The model under review builds one solid part; all positions refer to its coordinate system, in mm. Give positions to 0.01 mm unless a question says otherwise; leave off trailing zeros. Write each loop counter-clockwise with the first axis right and the second up, starting at its lowest first coordinate (ties: lowest second). Pieces come first, ordered by that corner, then holes. Notation, with made-up numbers: (17.25, 0.5) -> (47.25, 0.5) arc R17 cw to (47.25, 13.5) -> close; hole circle Ø9 at (13.5, 22). An arc over 180 degrees is marked (long way). Use CSV: the item, a comma, the result in double quotes.
```python
from build123d import *

# Parameters (mm, degrees)
EXTRUDE_1_DEPTH     = 3
SKETCH_4_R          = 1.5
CUT_EXTRUDE_2_DEPTH = 5
SKETCH_6_R          = 1.5
CUT_EXTRUDE_4_DEPTH = 5
SKETCH_7_W          = 3
SKETCH_7_H          = 15
CUT_EXTRUDE_5_DEPTH = 10


with BuildPart() as part:
    # 草图2 → 凸台-拉伸1 (new body)
    with BuildSketch(Plane.XY):
        Polygon((-7.5, 56.5), (-7.5, 55.5), (7.5, 55.5), (7.5, 56.5), (12, 56.5), (12, 48.5), (100, 5), (100, -20), (-100, -20), (-100, 5), (-12, 48.5), (-12, 56.5), align=None)
    extrude(amount=EXTRUDE_1_DEPTH)

    # 草图4 → 切除-拉伸2 (cut)
    with BuildSketch(Plane.XY.offset(3)):
        with Locations((-5, -5)):
            Circle(SKETCH_4_R)
        with Locations((5, -5)):
            Circle(SKETCH_4_R)
        with Locations((-5, -15)):
            Circle(SKETCH_4_R)
        with Locations((5, -15)):
            Circle(SKETCH_4_R)
    extrude(amount=-CUT_EXTRUDE_2_DEPTH, mode=Mode.SUBTRACT)

    # 草图6 → 切除-拉伸4 (cut)
    with BuildSketch(Plane.XY.offset(3)):
        with Locations((-9, 45.5)):
            Circle(SKETCH_6_R)
        with Locations((9, 45.5)):
            Circle(SKETCH_6_R)
    extrude(amount=-CUT_EXTRUDE_4_DEPTH, mode=Mode.SUBTRACT)

    # 草图7 → 切除-拉伸5 (cut)
    with BuildSketch(Plane.XY.offset(3)):
        with Locations((-58.5, 9.5)):
            Rectangle(SKETCH_7_W, SKETCH_7_H)
        with Locations((58.5, 9.5)):
            Rectangle(SKETCH_7_W, SKETCH_7_H)
    extrude(amount=-CUT_EXTRUDE_5_DEPTH, mode=Mode.SUBTRACT)


solid = part.part
```
Q1. Consider section A-A (z = 1.9). State how many separate pieces and enclosed holes the cut face has, then the cut area to 3 significant figures.
Derived:
separate pieces,"1"
enclosed holes,"8"
area,"9,920 mm2"
Q2. Insertion check: pin 1 (1.8 mm diameter, centred on x = -9, y = 45.5, fed in from -Z); pin 2 (1.5 mm diameter, centred on x = -1.5, z = 1.5, fed in from +Y); pin 3 (1.5 mm diameter, centred on y = 8.5, z = 2, fed in from -X); pin 4 (1.5 mm diameter, centred on y = 51, z = 1, fed in from -X). Each pin has a flat end and moves straight along its axis. Give the tip position at first contact, or say it passes through.
Derived:
pin 1,"passes through"
pin 2,"stops at y = 55.5"
pin 3,"stops at x = -94.44"
pin 4,"stops at x = -12"
Q3. Consider section B-B (y = 13.5). Write out the cut boundary in (x, z).
Derived:
outline,"(-82.8, 0) -> (-60, 0) -> (-60, 3) -> (-82.8, 3) -> close; (-57, 0) -> (57, 0) -> (57, 3) -> (-57, 3) -> close; (60, 0) -> (82.8, 0) -> (82.8, 3) -> (60, 3) -> close"
Q4. Consider section C-C (x = 71.5). Write out the cut boundary in (y, z), then the cut area to 3 significant figures.
Derived:
outline,"(-20, 0) -> (19.09, 0) -> (19.09, 3) -> (-20, 3) -> close"
area,"117 mm2"
Q5. To check wall thickness, follow probe 1 along Y at (x, z) = (-5, 1.75); probe 2 along X at (y, z) = (4, 2); probe 3 along X at (y, z) = (-14, 1.6). State the ranges of each line that lie inside material, in increasing order.
Derived:
probe 1,"y = -20 to -16.5, -13.5 to -6.5, -3.5 to 55.5"
probe 2,"x = -100 to -60, -57 to 57, 60 to 100"
probe 3,"x = -100 to -6.12, -3.88 to 3.88, 6.12 to 100"
Q6. Consider section D-D (x = -74). Write out the cut boundary in (y, z).
Derived:
outline,"(-20, 0) -> (17.85, 0) -> (17.85, 3) -> (-20, 3) -> close"
